Model file for the job. Use its own axes, mm. A direction names the side the tool comes from. Round coordinates to 2 decimals unless told otherwise and drop trailing zeros. Order: outer loops, then holes, each group sorted by start corner. A loop starts at its lowest first (then second) coordinate and runs counter-clockwise, first axis right, second up. Notation, with made-up numbers: M 17,45 L 32,45 A19 ccw 32,70 Z; hole C 29,87 d3. An arc over 180 degrees is marked long. Return JSON: item names as keys, results as strings. Group by question number.
Item 1: Slice it at C-C on z = 232.5. Write the cut outline in (x, y) (3 decimals), then the cut area to 3 significant figures.
Item 2: Slice it at A-A on z = 130.5. Write the cut outline in (x, y) (3 decimals).
Item 3: Probe line 1 along Z through (x, y) = (50.5, 9.5); line 2 along Z through (x, y) = (-22.5, 43.5); line 3 along Z through (x, y) = (51.5, 59.5). List the from-to ranges inside material, lowest first.
Item 4: Slice it at D-D on z = 51.5. Write the cut outline in (x, y) (3 decimals), then the cut area to 3 significant figures.
Item 5: Pin check, flat tips, straight feed: pin 1 Ø6 at (x, z) = (64.5, 53) entering from -Y; pin 2 Ø6 at (x, y) = (47.5, 3) entering from -Z; pin 3 Ø2 at (x, y) = (57.5, 28) entering from +Z; pin 4 Ø8 at (x, z) = (44, 105.5) entering from +Y. Stop position of each tip, or through.
Item 6: Slice it at B-B on x = 0. Write the cut outline in (y, z), then the cut area to 3 significant figures.
Item 7: Which spindle directions (+Z, -Z, +X, -X, +Y, -Y) get a long thin tool onto all of the face, cutting with end or side? Do faces 4 (the face through (30.718, 51.448, 128.468)), 5 (the face through (-16.995, 29.435, 128.778)), 6 (the face through (38.6, 64.65, 56.02)), 7 (the face through (32.45, 54.34, 233.08)), 8 (the face through (40.36, 67.59, 133.85)). Say none if no direction does.
Item 8: Pull direction Y, two halves, no side cores. Call faces 1 (the face through (32.658, 54.697, 102.856)), 2 (the face through (15, 29, 254)), 3 (the face through (34, 0, 129)): pulls with the +Y half, pulls with the -Y half, needs draft (parallel to the pull), parting line crosses it, or undercut.
from build123d import *

# Parameters (mm, degrees)
F0_R     = 6.35
F1_DEPTH = 254
F3_ANGLE = -120


with BuildPart() as f1:
    # F0 (on Top) → F1 (new body)
    with BuildSketch(Plane.XY):
        Circle(F0_R)
    extrude(amount=F1_DEPTH)

    # F2 (on Front) → F3 (revolve)
    with BuildSketch(Plane.XZ):
        Polygon((63.292921, 254), (6.35, 254), (6.35, 0), (56.434337, 18.382614), (37.573218, 41.816123), (75.295448, 41.816123), (75.295448, 69.822021), (52.433491, 134.978592), (78.724734, 112.116635), (78.724734, 154.982805), (30.714633, 211.566135), (63.292921, 211.566135), align=None)
    revolve(axis=Axis((0, 0, 121.26141), (0, 0, -1)), revolution_arc=F3_ANGLE)


solid = f1.part
Output values:
{
 "1": {"outline": "M -31.646,54.813 L -3.175,5.499 A6.35 ccw long 6.35,0 L 63.293,0 A63.293 ccw Z", "area": "4,280 mm²"},
 "2": {"outline": "M -39.362,68.178 L -28.792,49.869 A57.584 cw 57.584,0 L 78.725,0 A78.725 ccw Z; M -27.002,46.77 L -3.175,5.499 A6.35 ccw long 6.35,0 L 54.005,0 A54.005 ccw Z"},
 "3": {"line 1": "16.53 to 24.66, 41.82 to 187.2, 211.57 to 254", "line 2": "15.64 to 27.65, 41.82 to 190.05, 211.57 to 254", "line 3": "112.14 to 155.02"},
 "4": {"outline": "M -37.648,65.208 L -3.175,5.499 A6.35 ccw long 6.35,0 L 75.295,0 A75.295 ccw Z", "area": "6,020 mm²"},
 "5": {"pin 1": "y = 0", "pin 2": "z = 14.04", "pin 3": "z = 254", "pin 4": "y = 48.85"},
 "6": {"outline": "M -6.35,0 L 6.35,0 L 56.43,18.38 L 37.57,41.82 L 75.3,41.82 L 75.3,69.82 L 52.43,134.98 L 78.72,112.12 L 78.72,154.98 L 30.71,211.57 L 63.29,211.57 L 63.29,254 L -6.35,254 Z", "area": "17,200 mm²"},
 "7": {"face 4": "none", "face 5": "+Z, -Z, -X", "face 6": "-Z, +Y", "face 7": "+Z, +Y", "face 8": "+Z, -Z, +Y"},
 "8": {"face 1": "undercut", "face 2": "needs draft", "face 3": "pulls with the -Y half"}
}
